Autodesk Inventor part; units mm, degrees
ref_plane "YZ Plane" through (0, 0, 0) normal (1, 0, 0) x (0, 1, 0)
ref_plane "XZ Plane" through (0, 0, 0) normal (0, 1, 0) x (-1, 0, 0)
ref_plane "XY Plane" through (0, 0, 0) normal (0, 0, 1) x (1, 0, 0)
sketch "Sketch1" plane through (0, 0, 0) normal (0, 0, 1) x (1, 0, 0)
  line L0 (169.4484, 80.0625) -> (169.4484, 105.4625)
  line L1 (169.4484, 105.4625) -> (166.2734, 105.4625)
  line L2 (-33.7516, 3.8625) -> (-33.7516, 105.4625)
  line L3 (-33.7516, 105.4625) -> (166.2734, 105.4625)
  line L4 (-33.7516, 105.4625) -> (118.6484, 105.4625)
  line L5 (118.6484, 105.4625) -> (118.6484, 80.0625)
  line L6 (118.6484, 80.0625) -> (-33.7516, 80.0625)
  line L7 (-33.7516, 80.0625) -> (-33.7516, 105.4625)
  line L8 (169.4484, 80.0625) -> (93.2484, 29.2625)
  line L9 (93.2484, 29.2625) -> (-33.7516, 3.8625)
  line L10 (92.0098, 32.2527) -> (166.2734, 81.7618)
  line L11 (166.2734, 102.2875) -> (166.2734, 102.2875)
  line L12 (166.2734, 81.7618) -> (166.2734, 105.4625)
  line L13 (-33.7516, 7.1687) -> (92.1562, 32.3503)
  line L14 (118.6484, 105.4625) -> (166.2734, 105.4625)
  line L15 (-33.7516, 7.1687) -> (-33.7516, 80.0625)
  point P0 (0, 0)
  point P1 (-21.0516, 92.7625)
  point P2 (4.3484, 92.7625)
  dimension "d2" = 25.4
  dimension "d3" = 203.2
  dimension "d4" = 76.2
  dimension "d15" = 12.7
  dimension "d16" = 25.4
  dimension "d17" = 12.7
  dimension "d25" = 152.4
  dimension "d26" = 25.4
  dimension "d29" = 50.8
  dimension "d30" = 76.2
  dimension "d31" = 3.175
extrude "Extrusion1" add sketch "Sketch1" against normal blind 203.2 contours L8 L9 L2 L13 L10 L12 L1 L0
extrude "Extrusion3" add sketch "Sketch1" against normal blind 3.175
sketch "Sketch2" plane through (0, 0, -203.2) normal (0, 0, -1) x (-1, 0, 0)
  line L0 (-169.4484, 80.0625) -> (-169.4484, 105.4625)
  line L1 (33.7516, 3.8625) -> (-169.4484, 80.0625)
  line L2 (-169.4484, 105.4625) -> (-166.2734, 105.4625)
  line L3 (-166.2734, 105.4625) -> (33.7516, 105.4625)
  line L4 (33.7516, 105.4625) -> (33.7516, 3.8625)
  line L5 (-93.2484, 29.2625) -> (-169.4484, 80.0625)
  line L6 (33.7516, 3.8625) -> (-93.2484, 29.2625)
  line L7 (-166.2734, 81.7618) -> (-166.2734, 105.4625)
  line L8 (-93.2484, 29.2625) -> (-169.4484, 80.0625)
  line L9 (-169.4484, 80.0625) -> (-169.4484, 105.4625)
  line L10 (-169.4484, 105.4625) -> (-166.2734, 105.4625)
  line L11 (-166.2734, 105.4625) -> (-166.2734, 81.7618)
  line L12 (-92.1562, 32.3503) -> (-166.2734, 81.7618)
  line L13 (33.7516, 3.8625) -> (-93.2484, 29.2625)
  line L14 (-92.1562, 32.3503) -> (33.7516, 7.1687)
  point P0 (0, 0)
extrude "Extrusion4" add sketch "Sketch2" against normal blind 3.175
hole "Hole1" at (-21.0516, 92.7625, 0) at (4.3484, 92.7625, 0) direction (0, 0, -1) diameter 6.35 depth 254 tip angle 118
extrude "Extrusion5" cut sketch "Sketch1" against normal blind 228.6 contours L5 L6 L2 L3
properties part number "ramp1"
Read the model definition and answer for the solid it produces. Units are mm, in the model's axes. A direction names the side the tool comes from. Round coordinates to 2 decimals unless told otherwise and drop trailing zeros. Write each loop counter-clockwise with the first axis right and the second up, starting at its lowest first coordinate (ties: lowest second). Pieces come first, ordered by that corner, then holes. Notation, with made-up numbers: M 71,29 L 96,29 A21 ccw 96,53 Z; hole C -18.5,-24.75 d8. An arc over 180 degrees is marked long. Use a Markdown table: item, result.
1) The part is cut by section B-B (y = 87.5). Write down the section's boundary in (x, z) (3 decimals).
Answers follow:
| item | result |
|---|---|
| outline | M 118.648,-203.2 L 169.448,-203.2 L 169.448,0 L 118.648,0 L 118.648,-3.175 L 166.273,-3.175 L 166.273,-200.025 L 118.648,-200.025 Z |
2) The part is cut by section A-A (z = -16). Write down the section's boundary in (x, y).
Answers follow:
| item | result |
|---|---|
| outline | M -33.75,3.86 L 93.25,29.26 L 169.45,80.06 L 169.45,105.46 L 166.27,105.46 L 166.27,81.76 L 92.16,32.35 L -33.75,7.17 Z |
3) Straight lines are drawn through the part: line 1 along Z through (x, y) = (8.5, 50) (3 decimals); line 2 along X through (y, z) = (84.5, -170.5); line 3 along X through (y, z) = (77.5, -45.5). For each, find the intervals that lie inside material, in ascending order. Write a range as [from, to].
Answers follow:
| item | result |
|---|---|
| line 1 | z = [-203.2, -200.025], [-3.175, 0] |
| line 2 | x = [166.27, 169.45] |
| line 3 | x = [159.88, 165.6] |
4) A tool of negligible diameter and unlimited length cuts with its end or side. For faces 4 (the flat face through (45, 57, -200.025)), 5 (the flat face through (44, 55, 0)), from which of +Z, -Z, +X, -X, +Y, -Y can it reach the whole face along a straight path? Write none if from no direction.
Answers follow:
| item | result |
|---|---|
| face 4 | -X, +Y |
| face 5 | +Z, +X, -X, +Y, -Y |
5) Flat-ended cylindrical pins translate along their axes: pin 1 (19 mm diameter, centred on y = 93, z = -93, fed in from -X); pin 2 (8 mm diameter, centred on x = -0.5, z = -128, fed in from -Y); pin 3 (2.5 mm diameter, centred on y = 87.5, z = -1, fed in from -X). Find the tip coordinate at first contact, or state that the pin passes through.
Answers follow:
| item | result |
|---|---|
| pin 1 | stops at x = 166.27 |
| pin 2 | stops at y = 9.71 |
| pin 3 | stops at x = 118.65 |
6) For a pull along Z with two mould halves and no side action, classify faces 1 (the flat face through (44, 55, -203.2)), 2 (the flat face through (131.882, 55.018, -100.178)), 3 (the flat face through (28.321, 19.583, -100.222)) as pulls with the +Z half, pulls with the -Z half, needs draft (parallel to the pull), parting line crosses it, or undercut.
Answers follow:
| item | result |
|---|---|
| face 1 | pulls with the -Z half |
| face 2 | needs draft |
| face 3 | undercut |
